```python
from build123d import *

# Parameters (mm, degrees)
SKETCH1_R           = 2.1
SKETCH1_R_2         = 1.5
SKETCH1_R_3         = 3
SKETCH1_R_4         = 19
BOSS_EXTRUDE1_DEPTH = 4
BOSS_EXTRUDE2_DEPTH = 2
FILLET1_R           = 10
SKETCH1_4_R         = 3
BOSS_EXTRUDE3_DEPTH = 6.9
FILLET2_R           = 3


with BuildPart() as part:
    # Sketch1 → Boss-Extrude1 (new body)
    with BuildSketch(Plane(origin=(0, 0, 0), x_dir=(1, 0, 0), z_dir=(0, 1, 0))):
        with BuildLine():
            ThreePointArc((-18.439088915, -31.5), (25.809397513, 25.809397513), (-31.5, -18.439088915))
            Line((-31.5, -18.439088915), (-31.5, -31.5))
            Line((-31.5, -31.5), (-18.439088915, -31.5))
        make_face()
        with Locations(Location((-28.135778823, -21.064711012, 0), (0, 0, 270))):
            Circle(SKETCH1_R, mode=Mode.SUBTRACT)
        with Locations(Location((-21.064711012, -28.135778823, 0), (0, 0, 270))):
            Circle(SKETCH1_R, mode=Mode.SUBTRACT)
        with Locations(Location((0, -31.5, 0), (0, 0, 270))):
            Circle(SKETCH1_R_2, mode=Mode.SUBTRACT)
        with Locations(Location((0, -25.25, 0), (0, 0, 270))):
            Circle(SKETCH1_R_3, mode=Mode.SUBTRACT)
        with Locations(Location((-31.5, 0, 0), (0, 0, 270))):
            Circle(SKETCH1_R_2, mode=Mode.SUBTRACT)
        with Locations(Location((-25.25, 0, 0), (0, 0, 270))):
            Circle(SKETCH1_R_3, mode=Mode.SUBTRACT)
        with Locations(Location((0, 0, 0), (0, 0, 270))):
            Circle(SKETCH1_R_4, mode=Mode.SUBTRACT)
        with Locations(Location((25.25, 0, 0), (0, 0, 270))):
            Circle(SKETCH1_R_3, mode=Mode.SUBTRACT)
        with Locations(Location((31.5, 0, 0), (0, 0, 270))):
            Circle(SKETCH1_R_2, mode=Mode.SUBTRACT)
        with Locations(Location((0, 25.25, 0), (0, 0, 270))):
            Circle(SKETCH1_R_3, mode=Mode.SUBTRACT)
        with Locations(Location((0, 31.5, 0), (0, 0, 270))):
            Circle(SKETCH1_R_2, mode=Mode.SUBTRACT)
    extrude(amount=BOSS_EXTRUDE1_DEPTH)

    # Sketch1<3> → Boss-Extrude2 (add)
    with BuildSketch(Plane(origin=(0, 0, 0), x_dir=(1, 0, 0), z_dir=(0, 1, 0))):
        with BuildLine():
            ThreePointArc((0, 19), (-17.553711118, 7.270985215), (-13.435028843, -13.435028843))
            ThreePointArc((-13.435028843, -13.435028843), (7.270985215, -17.553711118), (19, 0))
            ThreePointArc((19, 0), (13.435028843, 13.435028843), (0, 19))
        make_face()
        with BuildLine():
            ThreePointArc((-3.535533906, -3.535533906), (-3.535533906, 3.535533906), (3.535533906, 3.535533906))
            ThreePointArc((3.535533906, 3.535533906), (4.619397663, 1.913417162), (5, 0))
            ThreePointArc((5, 0), (1.913417162, -4.619397663), (-3.535533906, -3.535533906))
        make_face(mode=Mode.SUBTRACT)
        with BuildLine():
            ThreePointArc((15.329967876, 6.158900064), (12.426332668, 4.218753046), (11.745043636, 7.643824305))
            ThreePointArc((11.745043636, 7.643824305), (14.033603084, 8.099047082), (15.329967876, 6.158900064))
        make_face(mode=Mode.SUBTRACT)
        with BuildLine():
            ThreePointArc((8.258900064, 13.229967876), (8.099047082, 12.426332668), (7.643824305, 11.745043636))
            ThreePointArc((7.643824305, 11.745043636), (4.218753046, 14.033603084), (8.258900064, 13.229967876))
        make_face(mode=Mode.SUBTRACT)
    extrude(amount=BOSS_EXTRUDE2_DEPTH)

    # Fillet1
    fillet1_edges = [part.edges().sort_by_distance(p)[0] for p in [
        (-31.5, 2, 31.5),
    ]]
    fillet(fillet1_edges, radius=FILLET1_R)

    # Sketch1<4> → Boss-Extrude3 (add)
    with BuildSketch(Plane(origin=(0, 0, 0), x_dir=(1, 0, 0), z_dir=(0, 1, 0))):
        with Locations(Location((0, 25.25, 0), (0, 0, 90))):
            Circle(SKETCH1_4_R)
        with Locations(Location((25.25, 0, 0), (0, 0, 90))):
            Circle(SKETCH1_4_R)
        with Locations(Location((0, -25.25, 0), (0, 0, 90))):
            Circle(SKETCH1_4_R)
        with Locations(Location((-25.25, 0, 0), (0, 0, 90))):
            Circle(SKETCH1_4_R)
    extrude(amount=BOSS_EXTRUDE3_DEPTH)

    # Fillet2
    # the kernel refuses this fillet: 3 mm, written as the material it takes off along each edge
    with BuildSketch(Plane(origin=(0, 6.9, -25.25), x_dir=(0, 0, -1), z_dir=(1, 0, 0))) as fillet2_piece_1:
        with BuildLine():
            CenterArc((0.00166713, -3), FILLET2_R, 1.910213172, 88.089786828)
            Line((0.00166713, 0), (0.00166713, 0.06))
            Line((0.00166713, 0.06), (3, 0.06))
            Line((3, 0.06), (3.06, 0))
            ThreePointArc((3.06, 0), (3.06, -1.45), (3.059966657, -2.898))
            Line((3.059966657, -2.898), (3, -2.9))
        make_face()
    revolve(axis=Axis((0, 6.9, -25.25), (0, 1, 0)), mode=Mode.SUBTRACT)
    with BuildSketch(Plane(origin=(-25.25, 6.9, 0), x_dir=(0, 0, -1), z_dir=(1, 0, 0))) as fillet2_piece_2:
        with BuildLine():
            CenterArc((0.00166713, -3), FILLET2_R, 1.910213172, 88.089786828)
            Line((0.00166713, 0), (0.00166713, 0.06))
            Line((0.00166713, 0.06), (3, 0.06))
            Line((3, 0.06), (3.06, 0))
            ThreePointArc((3.06, 0), (3.06, -1.45), (3.059966657, -2.898))
            Line((3.059966657, -2.898), (3, -2.9))
        make_face()
    revolve(axis=Axis((-25.25, 6.9, 0), (0, 1, 0)), mode=Mode.SUBTRACT)
    with BuildSketch(Plane(origin=(25.25, 6.9, 0), x_dir=(0, 0, -1), z_dir=(1, 0, 0))) as fillet2_piece_3:
        with BuildLine():
            CenterArc((0.00166713, -3), FILLET2_R, 1.910213172, 88.089786828)
            Line((0.00166713, 0), (0.00166713, 0.06))
            Line((0.00166713, 0.06), (3, 0.06))
            Line((3, 0.06), (3.06, 0))
            ThreePointArc((3.06, 0), (3.06, -1.45), (3.059966657, -2.898))
            Line((3.059966657, -2.898), (3, -2.9))
        make_face()
    revolve(axis=Axis((25.25, 6.9, 0), (0, 1, 0)), mode=Mode.SUBTRACT)
    with BuildSketch(Plane(origin=(0, 6.9, 25.25), x_dir=(0, 0, -1), z_dir=(1, 0, 0))) as fillet2_piece_4:
        with BuildLine():
            CenterArc((0.00166713, -3), FILLET2_R, 1.910213172, 88.089786828)
            Line((0.00166713, 0), (0.00166713, 0.06))
            Line((0.00166713, 0.06), (3, 0.06))
            Line((3, 0.06), (3.06, 0))
            ThreePointArc((3.06, 0), (3.06, -1.45), (3.059966657, -2.898))
            Line((3.059966657, -2.898), (3, -2.9))
        make_face()
    revolve(axis=Axis((0, 6.9, 25.25), (0, 1, 0)), mode=Mode.SUBTRACT)


solid = part.part
```
The listing builds one solid part. Answer for the finished solid, in the listing's coordinates (mm). A direction names the side the tool comes from. Give positions to 0.01 mm unless a question says otherwise; leave off trailing zeros. Order: outer loops, then holes, each group sorted by start corner. A loop starts at its lowest first (then second) coordinate and runs counter-clockwise, first axis right, second up.
Item 1: The part is cut by section A-A, the plane x = 31.5. Give the vertices of the cut face in (y, z), and give its area (3 significant figures).
From the geometry:
outline: (0, -18.44) - (4, -18.44) - (4, -1.5) - (0, -1.5) - close; (0, 1.5) - (4, 1.5) - (4, 18.44) - (0, 18.44) - close
area: 136 mm2
Item 2: The part is cut by section B-B, the plane z = 16. Give the vertices of the cut face in (x, y), and give its area (3 significant figures).
From the geometry:
outline: (-32.81, 0) - (32.81, 0) - (32.81, 4) - (10.25, 4) - (10.25, 2) - (-10.25, 2) - (-10.25, 4) - (-32.81, 4) - close
area: 221 mm2
Item 3: Given pin 1 Ø2.5 at (x, z) = (6.16, -13.23) entering from -Y; pin 2 Ø1.5 at (x, y) = (-20.5, 2.5) entering from +Z; pin 3 Ø1.5 at (y, z) = (1, -6.5) entering from -X; pin 4 Ø12 at (x, z) = (-20.5, -29) entering from +Y, each flat-ended and moving along its own axis, determine where each tip first touches the part or whether it passes through.
From the geometry:
pin 1: passes through
pin 2: stops at z = 31.5
pin 3: stops at x = -36.04
pin 4: stops at y = 4
Item 4: The part is cut by section C-C, the plane x = -10. Give the vertices of the cut face in (y, z), and give its area (3 significant figures).
From the geometry:
outline: (0, -35.1) - (4, -35.1) - (4, -16.16) - (2, -16.16) - (2, 16.16) - (4, 16.16) - (4, 35.1) - (0, 35.1) - close
area: 216 mm2
Item 5: Which of the six approach directions +Z, -Z, +X, -X, +Y, -Y give full straight-line access (tool end or side, diameter ignored) to faces 1 (the face through (-30.235, 1.972, 0.806)), 2 (the face through (-31.5, 2, 20)), 3 (the face through (16, 4, 16))?
From the geometry:
face 1: +Y, -Y
face 2: +Z, -X, +Y, -Y
face 3: +Y
Item 6: Find the intervals of material crossed by probe 1 along X at (y, z) = (2.65, -31.5); probe 2 along Y at (x, z) = (11, 28.5); probe 3 along X at (y, z) = (3.25, -6), in increasing order.
From the geometry:
probe 1: x = -18.44 to -1.5, 1.5 to 18.44
probe 2: y = 0 to 4
probe 3: x = -36 to -18.03, 18.03 to 36
